```python
from build123d import *

# Parameters (mm, degrees)
F0_W     = 12.446
F0_H     = 431.8
F0_R     = 3.175
F1_DEPTH = 12.7


with BuildPart() as f1:
    # F0 (on Top) → F1 (new body)
    with BuildSketch(Plane.XY):
        Polygon((602.978926, 190.381889), (-616.221074, 190.381889), (-1028.069377, -107.015111), (-616.221074, -404.412111), (602.978926, -404.412111), align=None)
        with Locations((234.867118, -112.431925)):
            Rectangle(F0_W, F0_H, mode=Mode.SUBTRACT)
        with Locations((-882.655084, -107.015111)):
            Circle(F0_R, mode=Mode.SUBTRACT)
    extrude(amount=F1_DEPTH)


solid = f1.part
```
Design review of the part built by this model. Coordinates are the model's own, in mm. Round coordinates to 2 decimals unless told otherwise and drop trailing zeros. Order: outer loops, then holes, each group sorted by start corner. A loop starts at its lowest first (then second) coordinate and runs counter-clockwise, first axis right, second up. Notation, with made-up numbers: M -11,-36 L 7,-36 A31 ccw 7,-4 Z; hole C 50,26 d1. An arc over 180 degrees is marked long. Put each result on its own line as item: value.
Q1. Consider section B-B (y = 54). State the section outline as (x, z) points.
Reported:
outline: M -805.09,0 L 228.64,0 L 228.64,12.7 L -805.09,12.7 Z; M 241.09,0 L 602.98,0 L 602.98,12.7 L 241.09,12.7 Z
Q2. Consider section A-A (z = 5.5). State the section outline as (x, y) points (3 decimals).
Reported:
outline: M -1028.069,-107.015 L -616.221,-404.412 L 602.979,-404.412 L 602.979,190.382 L -616.221,190.382 Z; hole C -882.655,-107.015 d6.35; hole M 228.644,-328.332 L 241.09,-328.332 L 241.09,103.468 L 228.644,103.468 Z
Q3. Insertion check: pin 1 Ø6 at (y, z) = (-169, 4) entering from -X; pin 2 Ø1.5 at (y, z) = (41.5, 2) entering from -X. Each pin has a flat end and moves straight along its axis. Give the tip position at first contact, or say it passes through.
Reported:
pin 1: x = -946.38
pin 2: x = -823.44
Q4. Consider section C-C (y = -165.5). State the section outline as (x, z) points, and give its area (3 significant figures).
Reported:
outline: M -947.08,0 L 228.64,0 L 228.64,12.7 L -947.08,12.7 Z; M 241.09,0 L 602.98,0 L 602.98,12.7 L 241.09,12.7 Z
area: 19,500 mm²
Q5. To check wall thickness, follow line 1 (X direction, y = -181, z = 10.5); line 2 (X direction, y = 41.5, z = 11); line 3 (X direction, y = -376, z = 10.5). State the ranges of each line that lie inside material, in increasing order.
Reported:
line 1: -925.61 to 228.64, 241.09 to 602.98
line 2: -822.4 to 228.64, 241.09 to 602.98
line 3: -655.57 to 602.98
Q6. Consider section D-D (x = -844). State the section outline as (y, z) points.
Reported:
outline: M -239.93,0 L 25.9,0 L 25.9,12.7 L -239.93,12.7 Z
